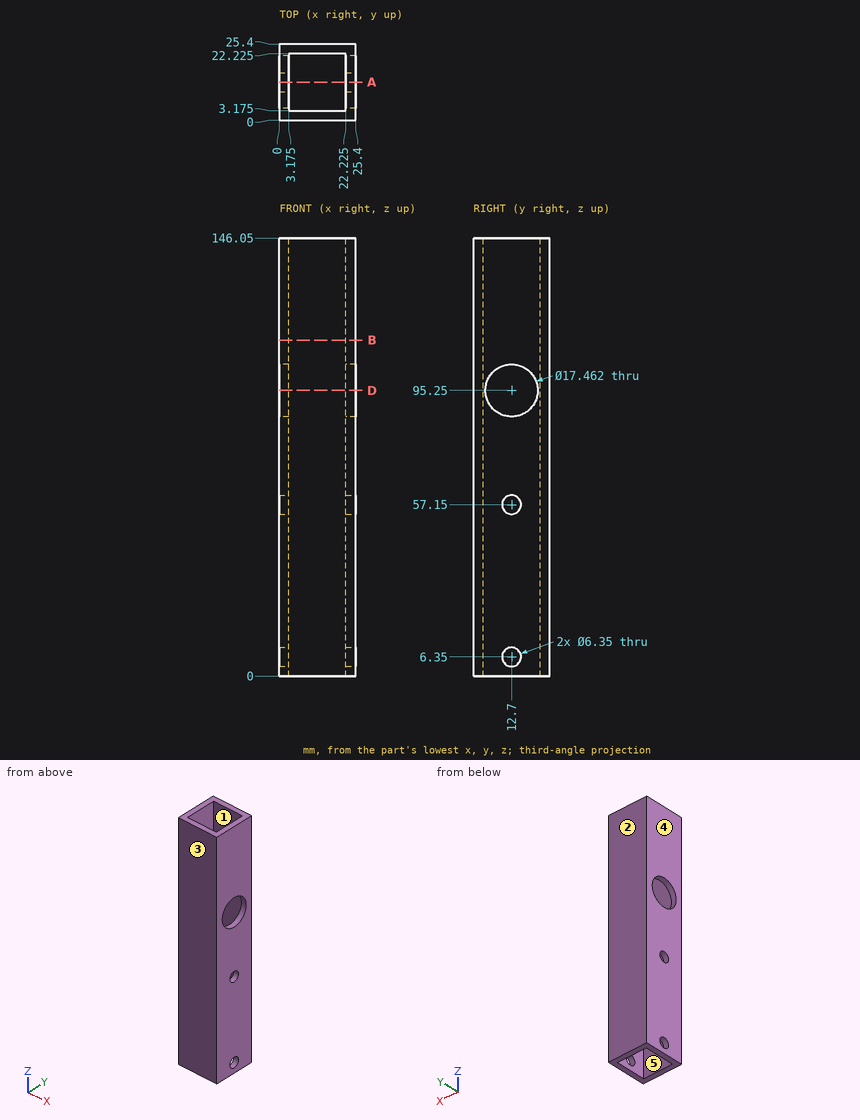
Here's the drawing with two shaded views (mm, measured from the low corner). I have some questions. A direction names the side the tool comes from. Round coordinates to 2 decimals unless told otherwise and drop trailing zeros. Order: outer loops, then holes, each group sorted by start corner. A loop starts at its lowest first (then second) coordinate and runs counter-clockwise, first axis right, second up. Notation, with made-up numbers: M 55.25,-2 L 79.25,-2 A19 cw 79.25,3 Z; hole C -14.5,26.25 d8. An arc over 180 degrees is marked long. Use CSV: the item, a comma, the result in double quotes.
1) I need wall thicknesses on line 1 along X through (y, z) = (8, 135.5) (1 decimal); line 2 along Y through (x, z) = (1.75, 57.15) (1 decimal). Which ranges of each line are inside material? Lowest first, please. Write a range as [from, to].
Taken from the geometry:
line 1,"[0, 3.2], [22.2, 25.4]"
line 2,"[0, 9.5], [15.9, 25.4]"
2) I'm going to push a flat-ended pin straight in: P1, Ø1, axis at x = 8, z = 96, coming from the -Y side. Where does the tip first touch, or does it pass through?
Taken from the geometry:
P1,"y = 0"
3) I want a section at A-A (y = 12.7). Count the separate pieces of the cut face and the enclosed holes in it.
Taken from the geometry:
separate pieces,"8"
enclosed holes,"0"
4) I want a section at B-B (z = 112). List the corners of the cut face in (x, y) for me (1 decimal).
Taken from the geometry:
outline,"M 0,0 L 25.4,0 L 25.4,25.4 L 0,25.4 Z; hole M 3.2,3.2 L 22.2,3.2 L 22.2,22.2 L 3.2,22.2 Z"
5) I want a section at D-D (z = 95.25). List the corners of the cut face in (x, y) for me (1 decimal), then the cut area to 3 significant figures.
Taken from the geometry:
outline,"M 0,0 L 25.4,0 L 25.4,4 L 22.2,4 L 22.2,3.2 L 3.2,3.2 L 3.2,4 L 0,4 Z; M 0,21.4 L 3.2,21.4 L 3.2,22.2 L 22.2,22.2 L 22.2,21.4 L 25.4,21.4 L 25.4,25.4 L 0,25.4 Z"
area,"171 mm^2"
6) On a 3-axis mill with a long thin cutter (end or side, diameter ignored), from which of +Z, -Z, +X, -X, +Y, -Y can I reach the whole of each face in a straight line? I mean the marked faces 1 and 2. Say none if no direction works.
Taken from the geometry:
face 1,"+Z, -Z"
face 2,"+Z, -Z, +X, -X, +Y"
7) If we mould it in two halves opening along X, with no side actions, what happens to the marked faces 3, 4 and 5? For each: pulls with the +X half, pulls with the -X half, needs draft (parallel to the pull), parting line crosses it, or undercut.
Taken from the geometry:
face 3,"needs draft"
face 4,"pulls with the -X half"
face 5,"undercut"
